Read the model definition and answer for the solid it produces. Units are mm, in the model's axes. Give positions to 0.01 mm unless a question says otherwise; leave off trailing zeros. Order: outer loops, then holes, each group sorted by start corner. A loop starts at its lowest first (then second) coordinate and runs counter-clockwise, first axis right, second up. Notation, with made-up numbers: (-15, 62) - (35, 62) arc R17 ccw to (35, 70) - close; hole circle Ø4 at (88.25, 37). An arc over 180 degrees is marked (long way). Return JSON: item names as keys, results as strings.
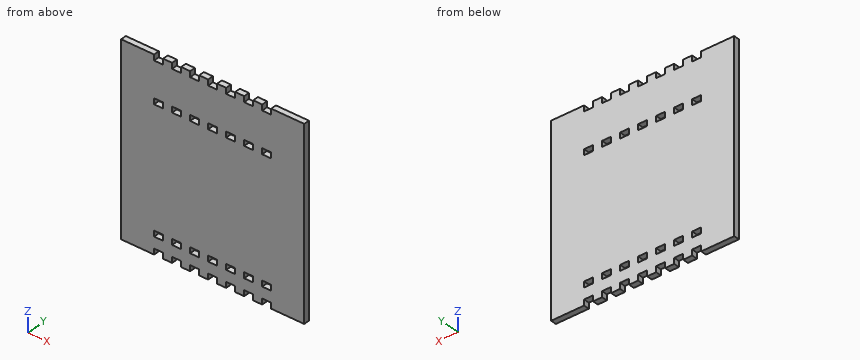
```python
from build123d import *

# Parameters (mm, degrees)
SKETCH1_W           = 5
SKETCH1_H           = 3.175
BOSS_EXTRUDE1_DEPTH = 3.175


with BuildPart() as part:
    # Sketch1 → Boss-Extrude1 (new body)
    with BuildSketch(Plane(origin=(0, 0, 0), x_dir=(1, 0, 0), z_dir=(0, 1, 0))):
        Polygon((-34.46085268, -90.343789474), (-34.46085268, -87.168789474), (-29.46085268, -87.168789474), (-29.46085268, -90.343789474), (-24.46085268, -90.343789474), (-24.46085268, -87.168789474), (-19.46085268, -87.168789474), (-19.46085268, -90.343789474), (-14.46085268, -90.343789474), (-14.46085268, -87.168789474), (-9.46085268, -87.168789474), (-9.46085268, -90.343789474), (-4.46085268, -90.343789474), (-4.46085268, -87.168789474), (0.53914732, -87.168789474), (0.53914732, -90.343789474), (5.53914732, -90.343789474), (5.53914732, -87.168789474), (10.53914732, -87.168789474), (10.53914732, -90.343789474), (15.53914732, -90.343789474), (15.53914732, -87.168789474), (20.53914732, -87.168789474), (20.53914732, -90.343789474), (25.53914732, -90.343789474), (25.53914732, -87.168789474), (30.53914732, -87.168789474), (30.53914732, -90.343789474), (48.83914732, -90.343789474), (48.83914732, 14.304210526), (30.53914732, 14.304210526), (30.53914732, 11.129210526), (25.53914732, 11.129210526), (25.53914732, 14.304210526), (20.53914732, 14.304210526), (20.53914732, 11.129210526), (15.53914732, 11.129210526), (15.53914732, 14.304210526), (10.53914732, 14.304210526), (10.53914732, 11.129210526), (5.53914732, 11.129210526), (5.53914732, 14.304210526), (0.53914732, 14.304210526), (0.53914732, 11.129210526), (-4.46085268, 11.129210526), (-4.46085268, 14.304210526), (-9.46085268, 14.304210526), (-9.46085268, 11.129210526), (-14.46085268, 11.129210526), (-14.46085268, 14.304210526), (-19.46085268, 14.304210526), (-19.46085268, 11.129210526), (-24.46085268, 11.129210526), (-24.46085268, 14.304210526), (-29.46085268, 14.304210526), (-29.46085268, 11.129210526), (-34.46085268, 11.129210526), (-34.46085268, 14.304210526), (-52.76085268, 14.304210526), (-52.76085268, -90.343789474), align=None)
        with Locations((-21.96085268, 3.318710526)):
            Rectangle(SKETCH1_W, SKETCH1_H, mode=Mode.SUBTRACT)
        with Locations((-31.96085268, 3.318710526)):
            Rectangle(SKETCH1_W, SKETCH1_H, mode=Mode.SUBTRACT)
        with Locations((-11.96085268, 3.318710526)):
            Rectangle(SKETCH1_W, SKETCH1_H, mode=Mode.SUBTRACT)
        with Locations((-1.96085268, 3.318710526)):
            Rectangle(SKETCH1_W, SKETCH1_H, mode=Mode.SUBTRACT)
        with Locations((8.03914732, 3.318710526)):
            Rectangle(SKETCH1_W, SKETCH1_H, mode=Mode.SUBTRACT)
        with Locations((18.03914732, 3.318710526)):
            Rectangle(SKETCH1_W, SKETCH1_H, mode=Mode.SUBTRACT)
        with Locations((28.03914732, 3.318710526)):
            Rectangle(SKETCH1_W, SKETCH1_H, mode=Mode.SUBTRACT)
        with Locations((-21.96085268, -65.882289474)):
            Rectangle(SKETCH1_W, SKETCH1_H, mode=Mode.SUBTRACT)
        with Locations((-31.96085268, -65.882289474)):
            Rectangle(SKETCH1_W, SKETCH1_H, mode=Mode.SUBTRACT)
        with Locations((-11.96085268, -65.882289474)):
            Rectangle(SKETCH1_W, SKETCH1_H, mode=Mode.SUBTRACT)
        with Locations((-1.96085268, -65.882289474)):
            Rectangle(SKETCH1_W, SKETCH1_H, mode=Mode.SUBTRACT)
        with Locations((8.03914732, -65.882289474)):
            Rectangle(SKETCH1_W, SKETCH1_H, mode=Mode.SUBTRACT)
        with Locations((18.03914732, -65.882289474)):
            Rectangle(SKETCH1_W, SKETCH1_H, mode=Mode.SUBTRACT)
        with Locations((28.03914732, -65.882289474)):
            Rectangle(SKETCH1_W, SKETCH1_H, mode=Mode.SUBTRACT)
    extrude(amount=BOSS_EXTRUDE1_DEPTH)


solid = part.part
```
Q1. A cutting plane is placed at B-B (y = 1). Give the number of separate pieces and of enclosed holes in the cut face, and give its area (3 significant figures).
Values:
{"separate pieces": "1", "enclosed holes": "14", "area": "10,200 mm²"}
Q2. Given pin 1 (1.6 mm diameter, centred on x = -31, y = 1, fed in from -Z); pin 2 (1.6 mm diameter, centred on x = 17.5, y = 1.5, fed in from +Z), each flat-ended and moving along its own axis, determine where each tip first touches the part or whether it passes through.
Values:
{"pin 1": "stops at z = -11.13", "pin 2": "stops at z = 87.17"}
Q3. A cutting plane is placed at A-A (x = 28.5). Write down the section's boundary in (y, z) (3 decimals), and give its area (3 significant figures).
Values:
{"outline": "(0, -11.129) - (3.175, -11.129) - (3.175, -4.906) - (0, -4.906) - close; (0, -1.731) - (3.175, -1.731) - (3.175, 64.295) - (0, 64.295) - close; (0, 67.47) - (3.175, 67.47) - (3.175, 87.169) - (0, 87.169) - close", "area": "292 mm²"}
Q4. Consider L1, parallel to Z at x = 20, y = 1.95. Determine where the line is inside the solid, lowest interval first.
Values:
{"L1": "z = -11.13 to -4.91, -1.73 to 64.29, 67.47 to 87.17"}
